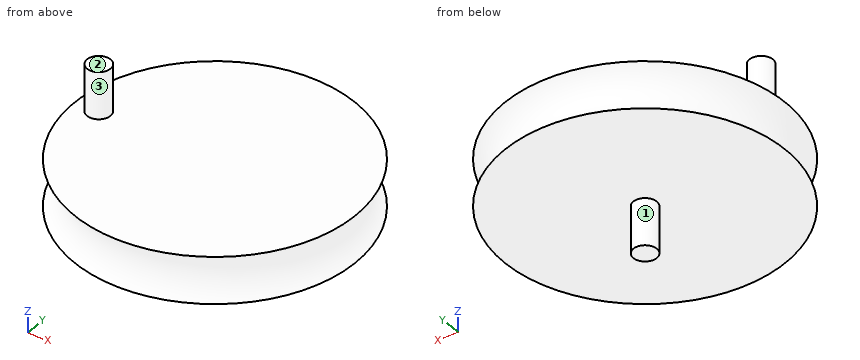
from build123d import *

# Parameters (mm, degrees)
F2_R     = 5
F3_DEPTH = 20
F4_R     = 5
F5_DEPTH = 30


with BuildPart() as f1:
    # F0 (on Front) → F1 (revolve)
    with BuildSketch(Plane.XZ):
        with BuildLine():
            Line((0, 70), (0, 0))
            Line((0, 0), (5, 0))
            Line((5, 0), (5, 20))
            Line((5, 20), (60, 20))
            ThreePointArc((60, 20), (54.662927, 30), (60, 40))
            Line((60, 40), (5, 40))
            Line((5, 40), (5, 70))
            Line((5, 70), (0, 70))
        make_face()
    revolve(axis=Axis((0, 0, 35), (0, 0, 1)))

    # F2 (on face) → F3 (join)
    with BuildSketch(Plane.XY.offset(40)):
        with Locations((-50, 0)):
            Circle(F2_R)
    extrude(amount=F3_DEPTH)

    # F4 (on face) → F5 (cut)
    with BuildSketch(Plane.XY.offset(70)):
        Circle(F4_R)
    extrude(amount=-F5_DEPTH, mode=Mode.SUBTRACT)


solid = f1.part
Could you check a few things on this model? Use its own coordinates, in mm. Face numbers are marked on the shaded views. A direction names the side the tool comes from. Round coordinates to 2 decimals unless told otherwise and drop trailing zeros. Order: outer loops, then holes, each group sorted by start corner. A loop starts at its lowest first (then second) coordinate and runs counter-clockwise, first axis right, second up.
(1) Please list where these lines run through material, in increasing order: line 1 along Z through (x, y) = (-4, -8.5); line 2 along Y through (x, z) = (44, 33); line 3 along Y through (x, z) = (-25, 26).
Response values:
line 1: z = 20 to 40
line 2: y = -33.07 to 33.07
line 3: y = -49.38 to 49.38
(2) Imagine slicing it at A-A (x = 0). Write out the boundary of the cut face in (y, z), plus the area to 3 significant figures.
Response values:
outline: (-60, 20) - (-5, 20) - (-5, 0) - (5, 0) - (5, 20) - (60, 20) arc R12.04 cw to (60, 40) - (-60, 40) arc R12.04 cw to start
area: 2,450 mm2
(3) I'm going to push flat-ended pins straight in: pin 1 (10 mm diameter, centred on x = -48, y = 3.5, fed in from -Z); pin 2 (1 mm diameter, centred on x = -30.5, y = 44.5, fed in from +Z); pin 3 (5 mm diameter, centred on y = 27, z = 18, fed in from +X). Where does each tip first touch, or does it pass through?
Response values:
pin 1: stops at z = 20
pin 2: stops at z = 40
pin 3: stops at x = 54.31
(4) Imagine slicing it at C-C (z = 18.5). Write out the boundary of the cut face in (x, y), plus the area to 3 significant figures.
Response values:
outline: circle Ø10 at (0, 0)
area: 78.5 mm2
(5) Imagine slicing it at B-B (y = 0). Write out the boundary of the cut face in (x, z), plus the area to 3 significant figures.
Response values:
outline: (-60, 20) - (-5, 20) - (-5, 0) - (5, 0) - (5, 20) - (60, 20) arc R12.04 cw to (60, 40) - (-45, 40) - (-45, 60) - (-55, 60) - (-55, 40) - (-60, 40) arc R12.04 cw to start
area: 2,650 mm2
(6) Which directions (+Z, -Z, +X, -X, +Y, -Y) give clear straight access to the entire face, cutting with the end or side of a thin tool? Please do the marked faces 1, 2 and 3.
Response values:
face 1: -Z
face 2: +Z, +X, -X, +Y, -Y
face 3: +Z
